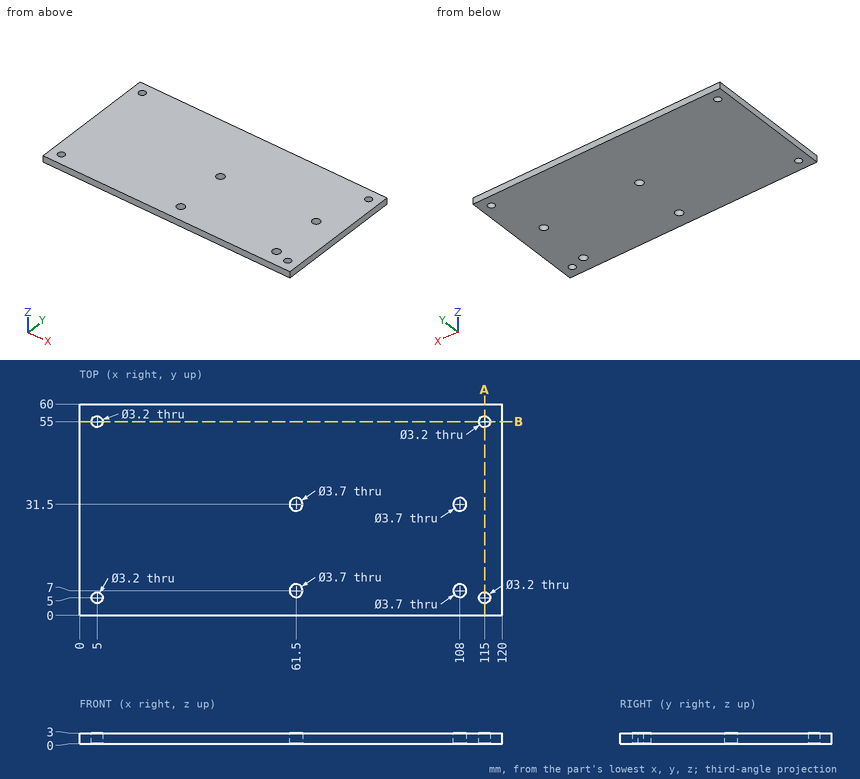
Here's the drawing with two shaded views (mm, measured from the low corner). I have some questions. Give positions to 0.01 mm unless a question says otherwise; leave off trailing zeros. Loops run counter-clockwise (first coordinate to the right, second up) from the corner with the lowest first, then second, coordinate; pieces in that order, holes last. Notation, with made-up numbers: M 3,83 L 28,83 A24 cw 28,97 Z; hole C 35,-13.75 d2. An arc over 180 degrees is marked long. One line per item, written item: value. Start each with the question number.
1) If we section it at B-B, the plane y = 55: Write out the boundary of the cut face in (x, z), and give its area (3 significant figures).
2) If we section it at A-A, the plane x = 115: Write out the boundary of the cut face in (y, z).
3) If I drill on line 1 (Y direction, x = 5, z = 1.1), over which ranges is the centre line in solid material (lowest first)? Write a range as [from, to].
4) I'm going to push a flat-ended pin straight in: pin 1 (4.5 mm diameter, centred on x = 61.5, y = 31.5, fed in from -Z). Where does the tip first touch, or does it pass through?
Completed:
1. outline: M 0,0 L 3.4,0 L 3.4,3 L 0,3 Z; M 6.6,0 L 113.4,0 L 113.4,3 L 6.6,3 Z; M 116.6,0 L 120,0 L 120,3 L 116.6,3 Z
1. area: 341 mm^2
2. outline: M 0,0 L 3.4,0 L 3.4,3 L 0,3 Z; M 6.6,0 L 53.4,0 L 53.4,3 L 6.6,3 Z; M 56.6,0 L 60,0 L 60,3 L 56.6,3 Z
3. line 1: y = [0, 3.4], [6.6, 53.4], [56.6, 60]
4. pin 1: stops at z = 0
